Source: CAD feature listing. Evaluate the final solid. Frame: model axes, mm. Give positions to 0.01 mm unless a question says otherwise; leave off trailing zeros. Order: outer loops, then holes, each group sorted by start corner. A loop starts at its lowest first (then second) coordinate and runs counter-clockwise, first axis right, second up. Notation, with made-up numbers: M 83,22 L 120,22 A32 ccw 120,53 Z; hole C 55,66 d10. An arc over 180 degrees is marked long. Answer in a Markdown table with one row per item. Add a question column.
(1) Material intervals for line 1 along X through (y, z) = (-11, 1.05) (3 decimals); line 2 along Y through (x, z) = (-28.5, 2); line 3 along X through (y, z) = (-90, 2.6) (3 decimals), sorted ascending.
(2) Pin query (flat end, axial travel): P1, Ø1, axis at x = 0, y = 57, coming from the -Z side; P2, Ø1.5, axis at y = -18, z = 2, coming from the -X side (3 decimals); P3, Ø2, axis at x = 14.94, y = 31.03, coming from the -Z side; P4, Ø1.5, axis at x = -89.5, z = 1, coming from the -Y side. Return the tip coordinate at first contact, or that it passes through.
(3) Section query A-A, the plane z = 1.9. Count the separate pieces of the cut face and the enclosed holes in it, plus the area to 3 significant figures.
(4) Section query B-B, the plane x = -63.5. Return loops of the section in (y, z), plus the area to 3 significant figures.
(5) Section query C-C, the plane y = -97.5. Return loops of the section in (x, z).
Solid Edge part; units mm, degrees
sketch "Sketch1" plane through (0, 0, 0) normal (0, 0, 1) x (1, 0, 0)
  circle A0 centre (-38.075, 61.7203) radius 1.65
  circle A1 centre (16.915, 61.7203) radius 1.65
  line L0 (-95.035, 70.5303) -> (94.945, 70.5303)
  line L1 (94.945, 70.5303) -> (94.945, -98.4697)
  line L2 (94.945, -98.4697) -> (-95.035, -98.4697)
  line L3 (-95.035, -98.4697) -> (-95.035, 70.5303)
  circle A2 centre (16.915, -89.2797) radius 1.65
  circle A3 centre (-38.075, -89.2797) radius 1.65
extrude "Protrusion1" add sketch "Sketch1" along normal blind 3
sketch "Sketch2" plane through (-0.045, -13.9697, 3) normal (0, 0, 1) x (-1, 0, 0)
  circle A0 centre (-14.99, 45) radius 1.65
  circle A1 centre (20.01, 45) radius 1.65
  circle A2 centre (20.01, -45) radius 1.65
  circle A3 centre (-14.99, -45) radius 1.65
extrude "Cutout1" cut sketch "Sketch2" against normal up to next
sketch "Sketch3" plane through (-0.045, -13.9697, 3) normal (0, 0, 1) x (0, -1, 0)
  circle A0 centre (-18, -75.99) radius 1.6
  circle A1 centre (-18, -90.99) radius 1.6
  circle A2 centre (0, -75.99) radius 1.6
  circle A3 centre (18, -75.99) radius 1.6
  circle A4 centre (18, -90.99) radius 1.6
  line L0 (11, -82.99) -> (-11, -82.99)
  line L1 (-11, -82.99) -> (-11, -94.99)
  line L2 (11, -94.99) -> (-11, -94.99)
  line L3 (11, -82.99) -> (11, -94.99)
extrude "Cutout2" cut sketch "Sketch3" against normal up to next
sketch "Sketch4" plane through (-0.045, -13.9697, 3) normal (0, 0, 1) x (0, 1, 0)
  arc A0 (-88.423, 88.1951) -> (-104.5, 28.1951) centre (15.5, 28.1951) ccw
  line L0 (-104.5, 28.1951) -> (-104.5, -59.5584)
  arc A1 (-104.5, -59.5584) -> (-87.9484, -94.4252) centre (-59.5, -59.5584) ccw
  line L1 (-87.9484, -94.4252) -> (-87.4195, -94.8567)
  arc A2 (-58.9711, -104.99) -> (-87.4195, -94.8567) centre (-58.9711, -59.99) cw
  line L2 (58.9711, -104.99) -> (-58.9711, -104.99)
  arc A3 (58.9711, -104.99) -> (87.4195, -94.8567) centre (58.9711, -59.99) ccw
  line L3 (87.4195, -94.8567) -> (87.9484, -94.4252)
  arc A4 (104.5, -59.5584) -> (87.9484, -94.4252) centre (59.5, -59.5584) cw
  line L4 (104.5, -59.5584) -> (104.5, 0)
  line L5 (104.5, 28.1951) -> (104.5, 0)
  arc A5 (88.423, 88.1951) -> (104.5, 28.1951) centre (-15.5, 28.1951) cw
  line L6 (84.5, 94.99) -> (88.423, 88.1951)
  line L7 (84.5, -94.99) -> (84.5, 94.99)
  line L8 (-84.5, -94.99) -> (84.5, -94.99)
  line L9 (-84.5, 94.99) -> (-84.5, -94.99)
  line L10 (-84.5, 94.99) -> (-88.423, 88.1951)
extrude "ExtrudedProtrusion_2" add sketch "Sketch4" against normal blind 3
fillet "Round_3" radius 8 2 edges at (-95.035, 70.5303, 1.5) (-95.035, -98.4697, 1.5)
Values follow:
| question | item | result |
|---|---|---|
| 1 | line 1 | x = -83.035 to 104.945 |
| 1 | line 2 | y = -118.47 to 90.53 |
| 1 | line 3 | x = -95.035 to -39.559, -36.591 to 15.431, 18.399 to 101.586 |
| 2 | P1 | stops at z = 0 |
| 2 | P2 | stops at x = -83.035 |
| 2 | P3 | passes through |
| 2 | P4 | stops at y = -102.1 |
| 3 | separate pieces | 1 |
| 3 | enclosed holes | 13 |
| 3 | area | 39,700 mm² |
| 4 | outline | M -113.17,0 L 85.23,0 L 85.23,3 L -113.17,3 Z |
| 4 | area | 595 mm² |
| 5 | outline | M -94.15,0 L 97.65,0 L 97.65,3 L -94.15,3 Z |
